Autodesk Inventor part; units mm, degrees
ref_plane "YZ Plane" through (0, 0, 0) normal (1, 0, 0) x (0, 1, 0)
ref_plane "XZ Plane" through (0, 0, 0) normal (0, 1, 0) x (-1, 0, 0)
ref_plane "XY Plane" through (0, 0, 0) normal (0, 0, 1) x (1, 0, 0)
sketch "Sketch1" plane through (0, 0, 0) normal (0, 1, 0) x (-1, 0, 0)
  line L0 (0, 0) -> (-21.59, 0)
  line L1 (-21.59, 0) -> (-21.59, -25.4)
  line L2 (-21.59, -25.4) -> (0, -25.4)
  line L3 (0, -25.4) -> (0, 0)
  line L4 (0, -25.4) -> (3.175, -25.4)
  line L5 (3.175, -25.4) -> (3.175, 3.175)
  line L6 (3.175, 3.175) -> (0, 3.175)
  line L7 (0, 3.175) -> (0, -25.4)
  line L8 (-21.59, -25.4) -> (-24.765, -25.4)
  line L9 (-24.765, -25.4) -> (-24.765, 3.175)
  line L10 (-24.765, 3.175) -> (-21.59, 3.175)
  line L11 (-21.59, 3.175) -> (-21.59, -25.4)
  line L12 (-21.59, 3.175) -> (0, 3.175)
  line L13 (0, 3.175) -> (0, 0)
  line L14 (0, 0) -> (-21.59, 0)
  line L15 (-21.59, 0) -> (-21.59, 3.175)
  dimension "d0" = 21.59
  dimension "d1" = 25.4
  dimension "d2" = 3.175
  dimension "d3" = 28.575
  dimension "d4" = 3.175
extrude "Extrusion1" add sketch "Sketch1" along normal blind 38.1 contours L7 L6 L5 L4 L3 | L0 L11 L12 L7 | L1 L8 L9 L10 L11
sketch "Sketch2" plane through (21.59, 0, 0) normal (0, 0, -1) x (-1, 0, 0)
  line L0 (24.765, 38.1) -> (-3.175, 38.1)
  line L1 (10.795, 38.1) -> (10.795, 26.67)
  line L2 (10.795, 38.1) -> (22.225, 38.1) construction
  line L3 (24.765, 0) -> (-3.175, 0)
  line L4 (10.795, 0) -> (10.795, 11.43)
  line L5 (10.795, 0) -> (22.225, 0) construction
  circle A0 centre (10.795, 26.67) radius 2.159
  circle A1 centre (10.795, 11.43) radius 2.159
  point P0 (21.59, 0)
  dimension "d7" = 11.43
  dimension "d8" = 90
  dimension "d9" = 11.43
  dimension "d10" = 90
  dimension "d11" = 4.318
  dimension "d12" = 4.318
sketch "Sketch3" plane through (-3.175, 0, -25.4) normal (-1, 0, 0) x (0, 0, 1)
  line L0 (28.575, 38.1) -> (0, 38.1)
  line L1 (0, 38.1) -> (10.795, 38.1)
  line L2 (10.795, 38.1) -> (10.795, 28.575)
  line L3 (28.575, 0) -> (0, 0)
  line L4 (10.795, 0) -> (10.795, 9.525)
  line L5 (10.795, 0) -> (20.32, 0) construction
  circle A0 centre (10.795, 28.575) radius 1.524
  circle A1 centre (10.795, 9.525) radius 2.54
  point P0 (25.4, 0)
  dimension "d13" = 10.795
  dimension "d14" = 9.525
  dimension "d15" = 90
  dimension "d16" = 9.525
  dimension "d17" = 90
  dimension "d18" = 3.048
  dimension "d19" = 5.08
extrude "Extrusion2" cut sketch "Sketch2" against normal blind 38.1
extrude "Extrusion3" cut sketch "Sketch3" against normal blind 38.1
fillet "Fillet1" radius 1.524 7 edges at (-3.175, 19.05, 3.175) (0, 19.05, 0) (24.765, 19.05, -25.4) (21.59, 19.05, -25.4) (21.59, 19.05, 0) (0, 19.05, -25.4) (-3.175, 19.05, -25.4)
properties part number "Long Robotics Mount V2"
The model under review builds one solid part; all positions refer to its coordinate system, in mm. A direction names the side the tool comes from. Round coordinates to 2 decimals unless told otherwise and drop trailing zeros. Write each loop counter-clockwise with the first axis right and the second up, starting at its lowest first coordinate (ties: lowest second). Pieces come first, ordered by that corner, then holes.
(1) We need section C-C on y = 11.43. Give the boundary of the cut face in (x, z) (3 decimals), and give its area (3 significant figures).
(2) We need section A-A on z = -20.25. Give the boundary of the cut face in (x, y) (3 decimals), and give its area (3 significant figures).
(3) Machinability: for faces 4 (the flat face through (24.765, 19, -11)), 5 (the flat face through (0, 19, -13)), which of the approach directions +Z, -Z, +X, -X, +Y, -Y give a long, thin tool a straight path to every point of the face, cutting with its end or side? Answer none if there is none.
(4) Mouldability with a two-part tool opening along X and no side actions: class faces 1 (the flat face through (21.59, 19, -13)), 2 (the flat face through (13, 38.1, 1)), 3 (the cylindrical face through (-2.74, 19.317, 2.717)) as +X half, -X half, draft (parallel to the pull), parting line (faces both ways), or undercut.
(5) We need section D-D on y = 17. Give the boundary of the cut face in (x, z) (3 decimals), and give its area (3 significant figures).
(6) We need section B-B on x = 9.5. Give the boundary of the cut face in (y, z) (1 decimal).
(7) Wall thickness on L1, parallel to X at y = 27, z = -13.25 (3 decimals); L2, parallel to Y at x = 23.25, z = -14.5; L3, parallel to Z at x = 19, y = 8 (3 decimals): over which ranges is each line inside the solid? List them lowest first.
(8) Insertion check: pin 1 (4 mm diameter, centred on x = 15, y = 11.5, fed in from -Z); pin 2 (2.5 mm diameter, centred on x = 10.795, y = 26.67, fed in from +Z); pin 3 (6 mm diameter, centred on x = 2, y = 19.5, fed in from -Z). Each pin has a flat end and moves straight along its axis. Give the tip position at first contact, or say it passes through.
Findings below:
1. outline: (-3.175, -23.876) arc R1.524 ccw to (-1.651, -25.4) - (-1.524, -25.4) arc R1.524 ccw to (0, -23.876) - (0, -16.285) - (-3.175, -16.285) - close; (-3.175, -12.925) - (0, -12.925) - (0, -1.524) arc R1.524 cw to (1.524, 0) - (8.636, 0) - (8.636, 3.175) - (-1.651, 3.175) arc R1.524 ccw to (-3.175, 1.651) - close; (12.954, 0) - (20.066, 0) arc R1.524 cw to (21.59, -1.524) - (21.59, -12.925) - (24.765, -12.925) - (24.765, 3.175) - (12.954, 3.175) - close; (21.59, -23.876) arc R1.524 ccw to (23.114, -25.4) - (23.241, -25.4) arc R1.524 ccw to (24.765, -23.876) - (24.765, -16.285) - (21.59, -16.285) - close
1. area: 213 mm2
2. outline: (-3.175, 0) - (0, 0) - (0, 38.1) - (-3.175, 38.1) - close; (21.59, 0) - (24.765, 0) - (24.765, 38.1) - (21.59, 38.1) - close
2. area: 242 mm2
3. face 4: +Z, -Z, +X, +Y, -Y
3. face 5: -Z, +Y, -Y
4. face 1: undercut
4. face 2: draft
4. face 3: -X half
5. outline: (-3.175, -23.876) arc R1.524 ccw to (-1.651, -25.4) - (-1.524, -25.4) arc R1.524 ccw to (0, -23.876) - (0, -1.524) arc R1.524 cw to (1.524, 0) - (20.066, 0) arc R1.524 cw to (21.59, -1.524) - (21.59, -23.876) arc R1.524 ccw to (23.114, -25.4) - (23.241, -25.4) arc R1.524 ccw to (24.765, -23.876) - (24.765, 3.175) - (-1.651, 3.175) arc R1.524 ccw to (-3.175, 1.651) - close
5. area: 249 mm2
6. outline: (0, 0) - (9.7, 0) - (9.7, 3.2) - (0, 3.2) - close; (13.2, 0) - (24.9, 0) - (24.9, 3.2) - (13.2, 3.2) - close; (28.4, 0) - (38.1, 0) - (38.1, 3.2) - (28.4, 3.2) - close
7. L1: x = -3.175 to 0, 21.59 to 24.765
7. L2: y = 0 to 6.99, 12.06 to 27.05, 30.1 to 38.1
7. L3: z = 0 to 3.175
8. pin 1: stops at z = 0
8. pin 2: passes through
8. pin 3: stops at z = -25.31
